from build123d import *

# Parameters (mm, degrees)
EXTRUDE1_DEPTH            = 6
SKETCH2_W                 = 44
SKETCH2_H                 = 44
EXTRUDE2_DEPTH            = 3
SKETCH4_R                 = 32.5
EXTRUDE3_DEPTH            = 17.5
SKETCH16_R                = 21
EXTRUDE7_DEPTH            = 12
SKETCH19_R                = 2.5
EXTRUDE8_DEPTH            = 24.5
LPATTERN1_COUNT           = 2
LPATTERN1_PITCH           = 56
LPATTERN2_COUNT           = 2
LPATTERN2_PITCH           = 56
LPATTERN2_COPY_1_SKETCH_R = 2.5
LPATTERN2_COPY_1_DEPTH    = 24.5
SKETCH20_R                = 12.5
EXTRUDE10_DEPTH           = 4


with BuildPart() as part:
    # Sketch1 → Extrude1 (new body)
    with BuildSketch(Plane(origin=(0, 0, 0), x_dir=(0, 0, -1), z_dir=(1, 0, 0))):
        Polygon((0, 68), (9, 77), (68, 77), (77, 68), (77, 9), (68, 0), (9, 0), (0, 9), align=None)
    extrude(amount=EXTRUDE1_DEPTH)

    # Sketch2 → Extrude2 (add)
    with BuildSketch(Plane(origin=(6, 0, 0), x_dir=(0, 0, -1), z_dir=(1, 0, 0))):
        with Locations((38.5, 38.5)):
            Rectangle(SKETCH2_W, SKETCH2_H)
    extrude(amount=EXTRUDE2_DEPTH)

    # Sketch4 → Extrude3 (add)
    with BuildSketch(Plane.ZY):
        with Locations((-38.5, 38.5)):
            Circle(SKETCH4_R)
    extrude(amount=EXTRUDE3_DEPTH)

    # Sketch16 → Extrude7 (cut)
    with BuildSketch(Plane.ZY.offset(17.5)):
        with Locations((-38.5, 38.5)):
            Circle(SKETCH16_R)
    extrude(amount=-EXTRUDE7_DEPTH, mode=Mode.SUBTRACT)

    # Sketch18 → Revolve2 (revolve)
    with BuildSketch(Plane.XZ.offset(-38.5)):
        Polygon((-5.5, -56.5), (-5.5, -59.5), (-17.5, -59.5), align=None)
    revolve(axis=Axis((9, 38.5, -38.5), (-1, 0, 0)))

    # Sketch19 → Extrude8 (cut, through all)
    with BuildSketch(Plane(origin=(6, 0, 0), x_dir=(0, 0, -1), z_dir=(1, 0, 0))):
        with Locations((10.5, 66.5)):
            Circle(SKETCH19_R)
    extrude8 = extrude(amount=-EXTRUDE8_DEPTH, mode=Mode.SUBTRACT)

    # LPattern1: Extrude8 ×2
    with Locations(*[(0, 0, -i * LPATTERN1_PITCH) for i in range(1, LPATTERN1_COUNT)]):
        add(extrude8, mode=Mode.SUBTRACT)

    # LPattern2: Extrude8 ×2
    with Locations(*[(0, -i * LPATTERN2_PITCH, 0) for i in range(1, LPATTERN2_COUNT)]):
        add(extrude8, mode=Mode.SUBTRACT)

    # LPattern2 copy 1 sketch → LPattern2 copy 1 (cut, through all)
    with BuildSketch(Plane(origin=(6, -56, -56), x_dir=(0, 0, -1), z_dir=(1, 0, 0))):
        with Locations((10.5, 66.5)):
            Circle(LPATTERN2_COPY_1_SKETCH_R)
    extrude(amount=-LPATTERN2_COPY_1_DEPTH, mode=Mode.SUBTRACT)

    # Sketch20 → Extrude10 (cut)
    with BuildSketch(Plane.ZY.offset(5.5)):
        with Locations((-38.5, 38.5)):
            Circle(SKETCH20_R)
    extrude(amount=-EXTRUDE10_DEPTH, mode=Mode.SUBTRACT)


solid = part.part
The listing builds one solid part. Answer for the finished solid, in the listing's coordinates (mm). A direction names the side the tool comes from. Round coordinates to 2 decimals unless told otherwise and drop trailing zeros. Order: outer loops, then holes, each group sorted by start corner. A loop starts at its lowest first (then second) coordinate and runs counter-clockwise, first axis right, second up. Notation, with made-up numbers: (63.5, 85) - (97.5, 85) arc R6 ccw to (97.5, 93) - close; hole circle Ø10 at (75, 74.5). An arc over 180 degrees is marked (long way). Write item = value, one per line. Start each with the question number.
1) Section B-B, the plane z = -10.5 is taken. Write down the section's boundary in (x, y).
2) Straight lines are drawn through the part: L1, parallel to Y at x = 3.4, z = -66.5; L2, parallel to Y at x = -2.4, z = -38.5; L3, parallel to Y at x = 7.5, z = -29.5. For each, find the intervals that lie inside material, in ascending order.
3) Given pin 1 (2.5 mm diameter, centred on x = 8, z = -46.5, fed in from +Y); pin 2 (2.5 mm diameter, centred on x = 7.5, y = 39.5, fed in from -Z); pin 3 (3.5 mm diameter, centred on x = 8, z = -30, fed in from -Y), each flat-ended and moving along its own axis, determine where each tip first touches the part or whether it passes through.
4) Section C-C, the plane x = -13.5 is taken. Write down the section's boundary in (y, z), plus the area to 3 significant figures.
5) For a pull along Y with two mould halves and no side action, classify faces 5 (the flat face through (-17.5, 39, -17)), 6 (the flat face through (-1.5, 39, -39)), 7 (the flat face through (3, 5, -73)) as released by +Y, released by -Y, zero draft, split by the parting line, or undercut.
6) Section D-D, the plane y = 38.5 is taken. Write down the section's boundary in (x, z).
7) For faces 1 (the flat face through (0, 39, -5)), 2 (the flat face through (7, 60.5, -38)), 3 (the flat face through (7, 38, -16.5)), 4 (the flat face through (7, 16.5, -38)), determine the directions among +Z, -Z, +X, -X, +Y, -Y from which every point of the face is accessible in a straight line to the end or side of a thin tool.
8) Section A-A, the plane y = 10.5 is taken. Write down the section's boundary in (x, z), plus the area to 4 significant figures.
Results list:
q1.outline = (-17.5, 22) - (0, 22) - (0, 13) - (6, 13) - (6, 64) - (0, 64) - (0, 55) - (-17.5, 55) - close; (0, 0) - (6, 0) - (6, 8) - (0, 8) - close; (0, 69) - (6, 69) - (6, 77) - (0, 77) - close
q2.L1 = 0 to 8, 13 to 64, 69 to 77
q2.L2 = 6 to 26, 51 to 71
q2.L3 = 16.5 to 60.5
q3.pin_1 = 60.5
q3.pin_2 = -60.5
q3.pin_3 = 16.5
q4.outline = circle Ø65 at (38.5, -38.5); hole circle Ø40 at (38.5, -38.5)
q4.area = 2,060 mm^2
q5.face_5 = zero draft
q5.face_6 = undercut
q5.face_7 = released by -Y
q6.outline = (-17.5, -71) - (0, -71) - (0, -77) - (6, -77) - (6, -60.5) - (9, -60.5) - (9, -16.5) - (6, -16.5) - (6, 0) - (0, 0) - (0, -6) - (-17.5, -6) - (-17.5, -17.5) - (-5.5, -20.5) - (-5.5, -26) - (-1.5, -26) - (-1.5, -51) - (-5.5, -51) - (-5.5, -56.5) - (-17.5, -59.5) - close
q7.face_1 = -X
q7.face_2 = +Z, -Z, +X, +Y
q7.face_3 = +Z, +X, +Y, -Y
q7.face_4 = +Z, -Z, +X, -Y
q8.outline = (-17.5, -55) - (0, -55) - (0, -64) - (6, -64) - (6, -13) - (0, -13) - (0, -22) - (-17.5, -22) - close; (0, -77) - (6, -77) - (6, -69) - (0, -69) - close; (0, -8) - (6, -8) - (6, 0) - (0, 0) - close
q8.area = 979.5 mm^2
